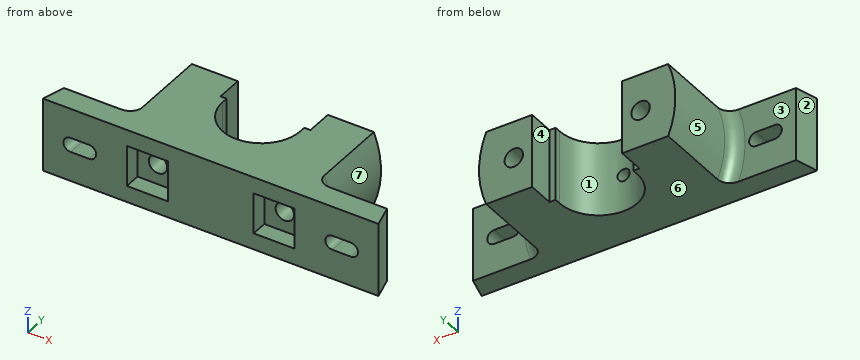
```python
from build123d import *

# Parameters (mm, degrees)
BOSS_EXTRUDE1_DEPTH       = 18
CUT_EXTRUDE1_DEPTH        = 43
CUT_EXTRUDE2_DEPTH        = 12
SKETCH6_W                 = 20
SKETCH6_H                 = 20
CUT_EXTRUDE3_DEPTH        = 8
SKETCH7_R                 = 4.5
CUT_EXTRUDE4_DEPTH        = 47
FILLET1_R                 = 6
F_6_0MM_DOWEL_HOLE1_D     = 6
F_6_0MM_DOWEL_HOLE1_DEPTH = 6
F_6_0MM_DOWEL_HOLE1_TIP   = 1.802581857


with BuildPart() as part:
    # Sketch1 → Boss-Extrude1 (new body, symmetric)
    with BuildSketch(Plane.XY):
        with BuildLine():
            Line((82, 0), (-82, 0))
            Line((-82, 0), (-79, 11))
            Line((-79, 11), (-50, 11))
            Line((-50, 11), (-50, 54))
            Line((-50, 54), (-22, 54))
            Line((-22, 54), (-22, 41))
            Line((-22, 41), (-19, 41))
            Line((-19, 41), (-19, 38))
            ThreePointArc((-19, 38), (0, 19), (19, 38))
            Line((19, 38), (19, 41))
            Line((19, 41), (22, 41))
            Line((22, 41), (22, 54))
            Line((22, 54), (50, 54))
            Line((50, 54), (50, 11))
            Line((50, 11), (79, 11))
            Line((79, 11), (82, 0))
        make_face()
    extrude(amount=BOSS_EXTRUDE1_DEPTH, both=True)

    # Sketch2 → Cut-Extrude1 (cut)
    with BuildSketch(Plane(origin=(0, 54, 0), x_dir=(1, 0, 0), z_dir=(0, 1, 0))):
        with BuildLine():
            Line((-44.497190923, -18), (-50, -18))
            Line((-50, -18), (-50, 18))
            Line((-50, 18), (-44.497190923, 18))
            ThreePointArc((-44.497190923, 18), (-48, 0), (-44.497190923, -18))
        make_face()
        with BuildLine():
            Line((50, 18), (44.497190923, 18))
            ThreePointArc((44.497190923, 18), (48, 0), (44.497190923, -18))
            Line((44.497190923, -18), (50, -18))
            Line((50, -18), (50, 18))
        make_face()
    extrude(amount=-CUT_EXTRUDE1_DEPTH, mode=Mode.SUBTRACT)

    # Sketch4 → Cut-Extrude2 (cut, through all)
    with BuildSketch(Plane(origin=(0, 11, 0), x_dir=(1, 0, 0), z_dir=(0, 1, 0))):
        with BuildLine():
            Line((-59.5, -3.5), (-68.5, -3.5))
            ThreePointArc((-68.5, -3.5), (-72, 0), (-68.5, 3.5))
            Line((-68.5, 3.5), (-59.5, 3.5))
            ThreePointArc((-59.5, 3.5), (-56, 0), (-59.5, -3.5))
        make_face()
    cut_extrude2 = extrude(amount=-CUT_EXTRUDE2_DEPTH, mode=Mode.SUBTRACT)

    # Sketch6 → Cut-Extrude3 (cut)
    with BuildSketch(Plane.XZ):
        with Locations((-31, 0)):
            Rectangle(SKETCH6_W, SKETCH6_H)
    cut_extrude3 = extrude(amount=-CUT_EXTRUDE3_DEPTH, mode=Mode.SUBTRACT)

    # Sketch7 → Cut-Extrude4 (cut, through all)
    with BuildSketch(Plane.XZ.offset(-8)):
        with Locations(Location((-31, 0, 0), (0, 0, 270))):  # turned: the seam where the file's is
            Circle(SKETCH7_R)
    cut_extrude4 = extrude(amount=-CUT_EXTRUDE4_DEPTH, mode=Mode.SUBTRACT)

    # Fillet1
    fillet1_edges = [part.edges().sort_by_distance(p)[0] for p in [
        (48, 11, 0),
        (-48, 11, 0),
    ]]
    fillet(fillet1_edges, radius=FILLET1_R)

    # Mirror6: Cut-Extrude2, Cut-Extrude3, Cut-Extrude4 across plane
    add(cut_extrude2.mirror(Plane(origin=(0, 0, 0), x_dir=(0, 0, 1), z_dir=(1, 0, 0))), mode=Mode.SUBTRACT)
    add(cut_extrude3.mirror(Plane(origin=(0, 0, 0), x_dir=(0, 0, 1), z_dir=(1, 0, 0))), mode=Mode.SUBTRACT)
    add(cut_extrude4.mirror(Plane(origin=(0, 0, 0), x_dir=(0, 0, 1), z_dir=(1, 0, 0))), mode=Mode.SUBTRACT)

    # Ø6.0mm Dowel Hole1
    with Locations(Plane(origin=(0, 19, 0), x_dir=(1, 0, 0), z_dir=(0, 1, 0))):
        with Locations((0, 0)):
            Hole(F_6_0MM_DOWEL_HOLE1_D / 2, depth=F_6_0MM_DOWEL_HOLE1_DEPTH)
            with Locations((0, 0, -(F_6_0MM_DOWEL_HOLE1_DEPTH + F_6_0MM_DOWEL_HOLE1_TIP / 2))):  # 118° drill point
                Cone(0, F_6_0MM_DOWEL_HOLE1_D / 2, F_6_0MM_DOWEL_HOLE1_TIP, mode=Mode.SUBTRACT)


solid = part.part
```
Verification items for the finished model (mm, model axes). Face numbers are marked on the shaded views. A direction names the side the tool comes from. Give positions to 0.01 mm unless a question says otherwise; leave off trailing zeros. Order: outer loops, then holes, each group sorted by start corner. A loop starts at its lowest first (then second) coordinate and runs counter-clockwise, first axis right, second up. Notation, with made-up numbers: M -23.5,46.5 L -1.5,46.5 A31 cw -1.5,77.5 Z; hole C 46.25,-23 d3. An arc over 180 degrees is marked long. Answer in a Markdown table with one row per item. Add a question column.
Item 1: Gauge pin test, flat ends, axial feed: pin 1 (4 mm diameter, centred on y = 4, z = 1.5, fed in from -X); pin 2 (1 mm diameter, centred on y = 30.5, z = 8, fed in from -X); pin 3 (4 mm diameter, centred on y = 15, z = -6, fed in from +X). Record the tip position at first contact, or that the pin passes through.
Item 2: Section check C-C, the plane x = -38. Enter the section's corners in (y, z), and give its area (3 significant figures).
Item 3: Scan lines: probe 1 along Z at (x, y) = (23, 7); probe 2 along Z at (x, y) = (31, 39); probe 3 along X at (y, z) = (23, -2). Record each from-to range of solid material in increasing order. Write a range as from..to.
Item 4: Section check B-B, the plane x = 31. Enter the section's corners in (y, z), and give its area (3 significant figures).
Item 5: Tool access check on the marked faces 4, 5, 6 and 7. Record the directions out of +Z, -Z, +X, -X, +Y, -Y that give a thin tool (end or side, any length) a straight path to the whole face; none if there is none.
Item 6: Section check A-A, the plane y = 43. Enter the section's corners in (x, z).
Item 7: Mould release check, pull along X, two halves, no side actions. Record for the marked faces 1, 2 and 3: released by +X, released by -X, zero draft, split by the parting line, or undercut.
Item 8: Section check D-D, the plane y = 36.5. Enter the section's corners in (x, z), and give its area (3 significant figures).
Filled sheet:
| question | item | result |
|---|---|---|
| 1 | pin 1 | stops at x = -81.45 |
| 1 | pin 2 | stops at x = -47.41 |
| 1 | pin 3 | stops at x = 49.18 |
| 2 | outline | M 0,-18 L 54,-18 L 54,18 L 0,18 L 0,10 L 8,10 L 8,-10 L 0,-10 Z |
| 2 | area | 1,780 mm^2 |
| 3 | probe 1 | z = -18..-10, 10..18 |
| 3 | probe 2 | z = -18..-4.5, 4.5..18 |
| 3 | probe 3 | x = -47.96..-35.03, -26.97..-11.66, 11.66..26.97, 35.03..47.96 |
| 4 | outline | M 0,-18 L 54,-18 L 54,-4.5 L 8,-4.5 L 8,-10 L 0,-10 Z; M 0,10 L 8,10 L 8,4.5 L 54,4.5 L 54,18 L 0,18 Z |
| 4 | area | 1,370 mm^2 |
| 5 | face 4 | +Z, -Z, +Y |
| 5 | face 5 | -X, +Y |
| 5 | face 6 | -Z, +X, -X, +Y, -Y |
| 5 | face 7 | +X, +Y |
| 6 | outline | M -44.5,-18 L -22,-18 L -22,18 L -44.5,18 A48 ccw Z; M 22,-18 L 44.5,-18 A48 ccw 44.5,18 L 22,18 Z; hole C -31,0 d9; hole C 31,0 d9 |
| 7 | face 1 | undercut |
| 7 | face 2 | released by -X |
| 7 | face 3 | zero draft |
| 8 | outline | M -44.5,-18 L -18.94,-18 L -18.94,18 L -44.5,18 A48 ccw Z; M 18.94,-18 L 44.5,-18 A48 ccw 44.5,18 L 18.94,18 Z; hole C -31,0 d9; hole C 31,0 d9 |
| 8 | area | 1,880 mm^2 |
